```python
from build123d import *

# Parameters (mm, degrees)
SKETCH1_W               = 180
SKETCH1_H               = 100
BOSS_EXTRUDE1_DEPTH     = 5
SKETCH2_W               = 160
SKETCH2_H               = 100
BOSS_EXTRUDE2_DEPTH     = 90
SKETCH3_R               = 2
CUT_EXTRUDE1_DEPTH      = 137.747943312
FILLET1_R               = 5
FILLET2_R               = 2
SKETCH4_W               = 65
SKETCH4_H               = 75
CUT_EXTRUDE2_DEPTH      = 85
FILLET3_R               = 10
CUT_EXTRUDE3_DEPTH      = 202.059692701
CUT_EXTRUDE3_DEPTH_BACK = 202.059692701
SKETCH5_W               = 60
SKETCH5_H               = 5


with BuildPart() as part:
    # Sketch1 → Boss-Extrude1 (new body)
    with BuildSketch(Plane(origin=(0, 0, 0), x_dir=(1, 0, 0), z_dir=(0, 1, 0))):
        Rectangle(SKETCH1_W, SKETCH1_H)
    extrude(amount=BOSS_EXTRUDE1_DEPTH)

    # Sketch2 → Boss-Extrude2 (add)
    with BuildSketch(Plane(origin=(0, 5, 0), x_dir=(1, 0, 0), z_dir=(0, 1, 0))):
        Rectangle(SKETCH2_W, SKETCH2_H)
    extrude(amount=BOSS_EXTRUDE2_DEPTH)

    # Sketch3 → Cut-Extrude1 (cut, through all)
    with BuildSketch(Plane(origin=(0, 5, 0), x_dir=(1, 0, 0), z_dir=(0, 1, 0))):
        with Locations(Location((-85, 30, 0), (0, 0, 270))):
            Circle(SKETCH3_R)
        with Locations(Location((85, 30, 0), (0, 0, 90))):
            Circle(SKETCH3_R)
        with Locations(Location((85, -30, 0), (0, 0, 270))):
            Circle(SKETCH3_R)
        with Locations(Location((-85, -30, 0), (0, 0, 90))):
            Circle(SKETCH3_R)
    extrude(amount=-CUT_EXTRUDE1_DEPTH, mode=Mode.SUBTRACT)

    # Fillet1
    fillet1_edges = [part.edges().sort_by_distance(p)[0] for p in [
        (-80, 50, -50),
        (-80, 50, 50),
        (80, 50, 50),
        (80, 50, -50),
        (-90, 2.5, -50),
        (90, 2.5, -50),
        (90, 2.5, 50),
        (-90, 2.5, 50),
    ]]
    fillet(fillet1_edges, radius=FILLET1_R)

    # Fillet2
    # the kernel refuses this fillet: 2 mm, written as the material it adds along each edge
    with BuildSketch(Plane(origin=(-80, 5, 45), x_dir=(0, 1, 0), z_dir=(0, 0, -1)), Plane(origin=(80, 5, -45), x_dir=(0, 1, 0), z_dir=(0, 0, 1))) as fillet2_piece_1:
        with BuildLine():
            CenterArc((FILLET2_R, -FILLET2_R), FILLET2_R, 90, 90)
            Line((0, -FILLET2_R), (0, 0))
            Line((0, 0), (FILLET2_R, 0))
        make_face()
    extrude(amount=90)
    with BuildSketch(Plane(origin=(-75, 5, -45), x_dir=(-1, 0, 0), z_dir=(0, 0, 1))) as fillet2_piece_2_section:
        with BuildLine():
            CenterArc((5 + FILLET2_R, -FILLET2_R), FILLET2_R, 90, 90)
            Line((5 + FILLET2_R, 0), (5, 0))
            Line((5, 0), (5, -FILLET2_R))
        make_face()
    fillet2_piece_2 = revolve(axis=Axis((-75, 5, -45), (0, -1, 0)), revolution_arc=147.318795695, mode=Mode.PRIVATE)
    fillet2_piece_2 = split(fillet2_piece_2, bisect_by=Plane(origin=(-78.61306887, 5.526930213, -50), z_dir=(0, 0, 1)), keep=Keep.TOP, mode=Mode.PRIVATE)
    add(fillet2_piece_2)
    with BuildSketch(Plane(origin=(75, 5, -45), x_dir=(1, 0, 0), z_dir=(0, 0, 1))) as fillet2_piece_3_section:
        with BuildLine():
            CenterArc((5 + FILLET2_R, FILLET2_R), FILLET2_R, 180, 90)
            Line((5 + FILLET2_R, 0), (5, 0))
            Line((5, 0), (5, FILLET2_R))
        make_face()
    fillet2_piece_3 = revolve(axis=Axis((75, 5, -45), (0, 1, 0)), revolution_arc=147.318795695, mode=Mode.PRIVATE)
    fillet2_piece_3 = split(fillet2_piece_3, bisect_by=Plane(origin=(78.613069351, 5.526929856, -50), z_dir=(0, 0, 1)), keep=Keep.TOP, mode=Mode.PRIVATE)
    add(fillet2_piece_3)
    with BuildSketch(Plane(origin=(-75, 5, 45), x_dir=(0.8416879607506224, 0, 0.5399642365263265), z_dir=(0.5399642365263265, 0, -0.8416879607506224))) as fillet2_piece_4_section:
        with BuildLine():
            CenterArc((5 + FILLET2_R, -FILLET2_R), FILLET2_R, 90, 90)
            Line((5, -FILLET2_R), (5, 0))
            Line((5, 0), (5 + FILLET2_R, 0))
        make_face()
    fillet2_piece_4 = revolve(axis=Axis((-75, 5, 45), (0, -1, 0)), revolution_arc=147.318795695, mode=Mode.PRIVATE)
    fillet2_piece_4 = split(fillet2_piece_4, bisect_by=Plane(origin=(-78.614624166, 5.52723882, 50), z_dir=(0, 0, -1)), keep=Keep.TOP, mode=Mode.PRIVATE)
    add(fillet2_piece_4)
    with BuildSketch(Plane(origin=(75, 5, 45), x_dir=(-0.8416879607506224, 0, 0.5399642365263265), z_dir=(-0.5399642365263265, 0, -0.8416879607506224))) as fillet2_piece_5_section:
        with BuildLine():
            CenterArc((5 + FILLET2_R, FILLET2_R), FILLET2_R, 180, 90)
            Line((5 + FILLET2_R, 0), (5, 0))
            Line((5, 0), (5, FILLET2_R))
        make_face()
    fillet2_piece_5 = revolve(axis=Axis((75, 5, 45), (0, 1, 0)), revolution_arc=147.318795695, mode=Mode.PRIVATE)
    fillet2_piece_5 = split(fillet2_piece_5, bisect_by=Plane(origin=(78.613068706, 5.526930627, 50), z_dir=(0, 0, -1)), keep=Keep.TOP, mode=Mode.PRIVATE)
    add(fillet2_piece_5)

    # Sketch4 → Cut-Extrude2 (cut)
    with BuildSketch(Plane(origin=(0, 95, 0), x_dir=(1, 0, 0), z_dir=(0, 1, 0))):
        with Locations((-37.5, 0)):
            Rectangle(SKETCH4_W, SKETCH4_H)
        with Locations((37.5, 0)):
            Rectangle(SKETCH4_W, SKETCH4_H)
    extrude(amount=-CUT_EXTRUDE2_DEPTH, mode=Mode.SUBTRACT)

    # Fillet3
    fillet3_edges = [part.edges().sort_by_distance(p)[0] for p in [
        (-70, 52.5, 37.5),
        (-70, 52.5, -37.5),
        (-5, 52.5, -37.5),
        (-5, 52.5, 37.5),
        (5, 52.5, 37.5),
        (5, 52.5, -37.5),
        (70, 52.5, -37.5),
        (70, 52.5, 37.5),
    ]]
    fillet(fillet3_edges, radius=FILLET3_R)

    # Sketch5 → Cut-Extrude3 (cut, two sides: drawn at the far end of the back side and taken through both)
    with BuildSketch(Plane.ZY.offset(80).offset(-CUT_EXTRUDE3_DEPTH_BACK)):
        with Locations((0, 82.5)):
            Rectangle(SKETCH5_W, SKETCH5_H)
    extrude(amount=CUT_EXTRUDE3_DEPTH + CUT_EXTRUDE3_DEPTH_BACK, mode=Mode.SUBTRACT)


solid = part.part
```
The model under review builds one solid part; all positions refer to its coordinate system, in mm. A direction names the side the tool comes from. Coordinates: 2 decimals unless noted, no trailing zeros. Loops run counter-clockwise (first coordinate to the right, second up) from the corner with the lowest first, then second, coordinate; pieces in that order, holes last. Notation, with made-up numbers: (36, 25.5) -> (52, 25.5) arc R21 cw to (52, 33.5) -> close; hole circle Ø8 at (2.5, 41). An arc over 180 degrees is marked (long way). Answer as CSV lines item,"result".
Item 1: For L1, parallel to X at y = 2.5, z = -30; L2, parallel to X at y = 44, z = -23.5; L3, parallel to Z at x = -29, y = 33.5, list the stretches that pass through material, from the lowest coordinate up.
Results below:
L1,"x = -90 to -87, -83 to 83, 87 to 90"
L2,"x = -80 to -70, -5 to 5, 70 to 80"
L3,"z = -50 to -37.5, 37.5 to 50"
Item 2: Insertion check: pin 1 (5 mm diameter, centred on x = -43, z = 32.5, fed in from +Y); pin 2 (3 mm diameter, centred on y = 92, z = 0, fed in from -X); pin 3 (5 mm diameter, centred on y = 88.5, z = -4.5, fed in from +X); pin 4 (3.5 mm diameter, centred on x = -85, z = 30, fed in from -Y). Each pin has a flat end and moves straight along its axis. Give the tip position at first contact, or say it passes through.
Results below:
pin 1,"stops at y = 10"
pin 2,"stops at x = -80"
pin 3,"stops at x = 80"
pin 4,"passes through"
Item 3: Take a section at C-C, the plane x = -48.5. State the section outline as (y, z) points, and give its area (4 significant figures).
Results below:
outline,"(0, -50) -> (95, -50) -> (95, -37.5) -> (10, -37.5) -> (10, 37.5) -> (95, 37.5) -> (95, 50) -> (0, 50) -> close"
area,"3,125 mm2"
Item 4: Draft analysis for pull direction X (two halves, no side actions). For faces 6 (the cylindrical face through (67.15, 51.9, -34.49)), 7 (the cylindrical face through (78, 52, 49)), 8 (the flat face through (-1, 47, 50)), state which applies: +X half, -X half, draft (parallel to the pull), parting line (faces both ways), or undercut.
Results below:
face 6,"undercut"
face 7,"+X half"
face 8,"draft"
Item 5: Machinability: for faces 1 (the cylindrical face through (83.314, 2.535, -31.075)), 2 (the flat face through (70, 90, 0)), 3 (the flat face through (-1, 48, -50)), 4 (the flat face through (75, 80, 0)), 5 (the cylindrical face through (78, 52, -49)), which of the approach directions +Z, -Z, +X, -X, +Y, -Y give a long, thin tool a straight path to every point of the face, cutting with its end or side? Answer none if there is none.
Results below:
face 1,"+Y, -Y"
face 2,"+Y"
face 3,"-Z, +X, -X, +Y, -Y"
face 4,"+X, -X"
face 5,"-Z, +X, +Y"
Item 6: Take a section at A-A, the plane z = -2. Count the separate pieces of the cut face and the enclosed holes in it, and give its area (3 significant figures).
Results below:
separate pieces,"4"
enclosed holes,"0"
area,"4,100 mm2"
Item 7: Take a section at B-B, the plane y = 76.5. State the section outline as (x, z) points.
Results below:
outline,"(-80, -45) arc R5 ccw to (-75, -50) -> (75, -50) arc R5 ccw to (80, -45) -> (80, 45) arc R5 ccw to (75, 50) -> (-75, 50) arc R5 ccw to (-80, 45) -> close; hole (-70, -27.5) arc R10 ccw to (-60, -37.5) -> (-15, -37.5) arc R10 ccw to (-5, -27.5) -> (-5, 27.5) arc R10 ccw to (-15, 37.5) -> (-60, 37.5) arc R10 ccw to (-70, 27.5) -> close; hole (5, -27.5) arc R10 ccw to (15, -37.5) -> (60, -37.5) arc R10 ccw to (70, -27.5) -> (70, 27.5) arc R10 ccw to (60, 37.5) -> (15, 37.5) arc R10 ccw to (5, 27.5) -> close"
